Geometry: final body of the model. Coordinates: model frame, mm. Face numbers are marked on the shaded views. A direction names the side the tool comes from. Give positions to 0.01 mm unless a question says otherwise; leave off trailing zeros. Order: outer loops, then holes, each group sorted by start corner. A loop starts at its lowest first (then second) coordinate and runs counter-clockwise, first axis right, second up. Notation, with made-up numbers: (-10, 36.25) -> (16, 36.25) arc R16 cw to (16, 58.25) -> close; hole circle Ø2 at (-23.75, 67). An arc over 180 degrees is marked (long way). Answer in a Markdown table with one row per item. Add a question column.
Q1. Cut plane C-C on y = -17. Return the cut outline in (x, z), and give its area (3 significant figures).
Q2. Contact query for flat-ended pins moving along their axis: P1, Ø5, axis at y = -20.5, z = -5.5, coming from the -X side; P2, Ø4, axis at y = -6.5, z = -1, coming from the +X side; P3, Ø2, axis at x = 21.5, y = -19, coming from the -Z side. Output: stop coordinate, or through.
Q3. Cut plane D-D on x = -6.5. Return the cut outline in (y, z).
Q4. Set-up query: the marked faces 1 and 2. Return all of +Z, -Z, +X, -X, +Y, -Y with unobstructed straight access to the full face (end or side cutting, diameter ignored); none if empty.
Q5. Line query: line 1 along Y through (x, z) = (-9, -5.75); line 2 along X through (y, z) = (-17, 0.75); line 3 along X through (y, z) = (-15.75, -1.5). Output: solid intervals per line, ascending. Write a range as from..to.
Q6. Cut plane A-A on z = 0. Return the cut outline in (x, y), and give its area (3 significant figures).
Q7. Cut plane B-B on x = 18.5. Return the cut outline in (y, z), and give its area (3 significant figures).
from build123d import *

# Parameters (mm, degrees)
F0_W     = 64.334008
F0_H     = 15.584806
F1_DEPTH = 2
F2_R     = 4.948824
F3_DEPTH = 25.2024
F4_R     = 5.08


with BuildPart() as f1:
    # F0 (on Front) → F1 (new body)
    with BuildSketch(Plane.XZ):
        Rectangle(F0_W, F0_H)
    extrude(amount=F1_DEPTH)

    # F2 (on face) → F3 (join)
    with BuildSketch(Plane.XZ.offset(2)):
        with Locations((17.712619, 0)):
            Circle(F2_R)
    extrude(amount=F3_DEPTH)

    # F4
    f4_edges = [f1.edges().sort_by_distance(p)[0] for p in [
        (-32.167004, -1, -7.792403),
        (-32.167004, -1, 7.792403),
        (32.167004, -1, -7.792403),
        (32.167004, -1, 7.792403),
    ]]
    fillet(f4_edges, radius=F4_R)


solid = f1.part
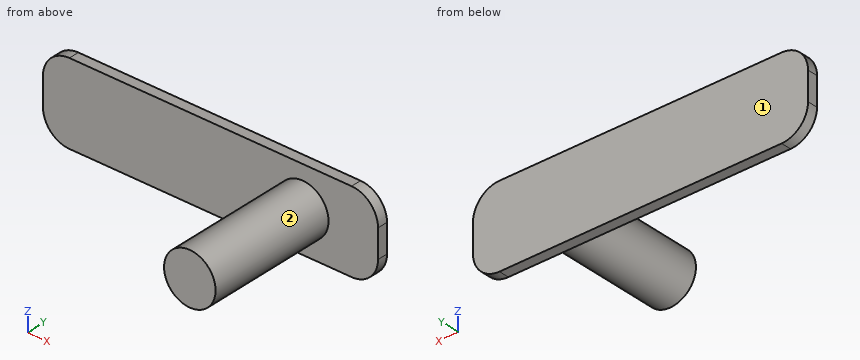
Completed:
| question | item | result |
|---|---|---|
| 1 | outline | circle Ø9.9 at (17.71, 0) |
| 1 | area | 76.9 mm² |
| 2 | P1 | stops at x = 13.78 |
| 2 | P2 | stops at x = 22.66 |
| 2 | P3 | stops at z = -4.09 |
| 3 | outline | (-2, -7.79) -> (0, -7.79) -> (0, 7.79) -> (-2, 7.79) -> close |
| 4 | face 1 | +Z, -Z, +X, -X, +Y |
| 4 | face 2 | -Y |
| 5 | line 1 | y = -2..0 |
| 5 | line 2 | x = 12.82..22.6 |
| 5 | line 3 | x = 13..22.43 |
| 6 | outline | (-32.17, -2) -> (12.76, -2) -> (12.76, -27.2) -> (22.66, -27.2) -> (22.66, -2) -> (32.17, -2) -> (32.17, 0) -> (-32.17, 0) -> close |
| 6 | area | 378 mm² |
| 7 | outline | (-27.2, -4.89) -> (-2, -4.89) -> (-2, -7.79) -> (0, -7.79) -> (0, 7.79) -> (-2, 7.79) -> (-2, 4.89) -> (-27.2, 4.89) -> close |
| 7 | area | 277 mm² |
